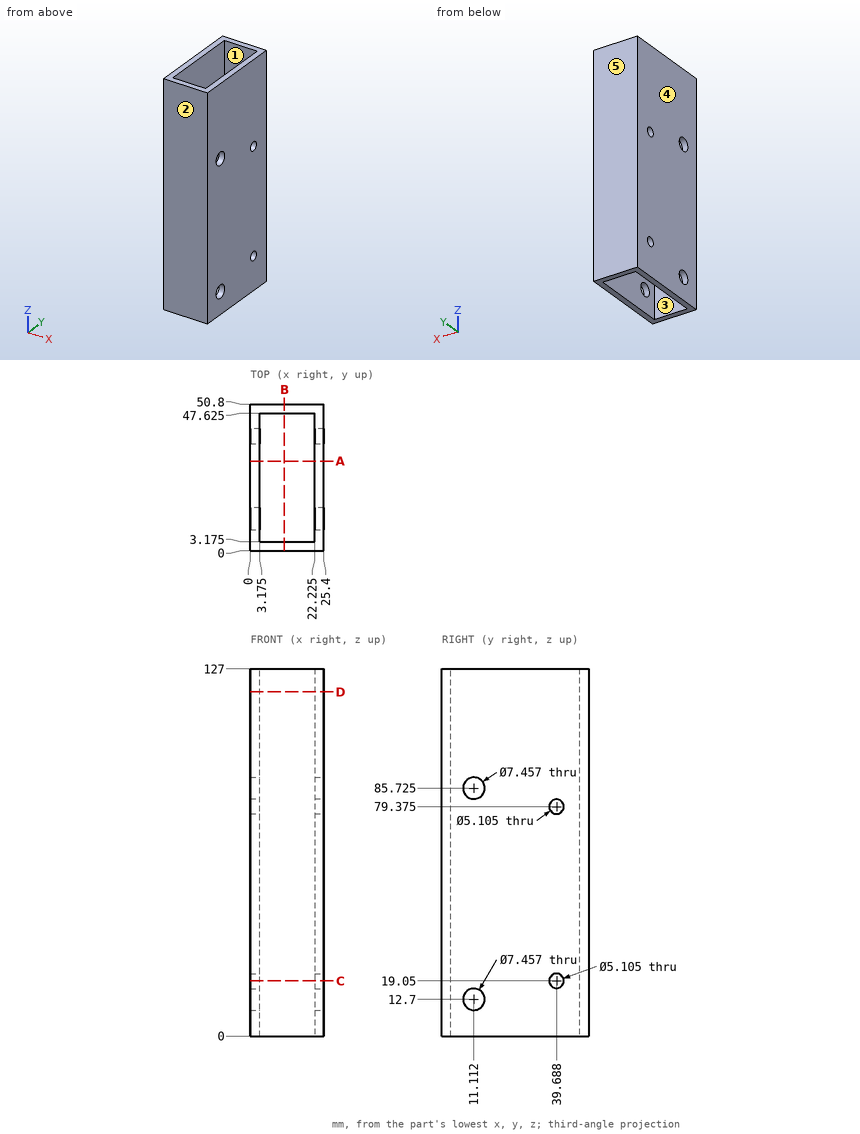
Source: three-view drawing plus pictorial views. Frame: mm from the lowest corner of the part. A direction names the side the tool comes from. Round coordinates to 2 decimals unless told otherwise and drop trailing zeros. Loops run counter-clockwise (first coordinate to the right, second up) from the corner with the lowest first, then second, coordinate; pieces in that order, holes last.
1. Section query A-A on y = 31. Output: boundary loops of the cut face in (x, z) (1 decimal).
2. Contact query for flat-ended pins moving along their axis: pin 1 (4.5 mm diameter, centred on y = 11.11, z = 85.72, fed in from +X); pin 2 (12 mm diameter, centred on x = 7.5, z = 35, fed in from -Y). Output: stop coordinate, or through.
3. Section query D-D on z = 119. Output: boundary loops of the cut face in (x, y) (1 decimal).
4. Mould query, pull axis X, two halves, no side actions, for the marked faces 3, 4 and 5. Classes: released by +X, released by -X, zero draft, split by the parting line, or undercut.
5. Ray query, L1, parallel to X at y = 31, z = 8 (1 decimal); L2, parallel to Y at x = 17.75, z = 112 (1 decimal). Return the intervals inside material, ascending.
6. Section query B-B on x = 11.75. Output: boundary loops of the cut face in (y, z) (1 decimal).
7. Access query for the marked faces 1 and 2. Directions: +Z, -Z, +X, -X, +Y, -Y. A direction counts if a zero-diameter tool reaches every point of the face in a straight line with its end or side. Return the directions, or none.
8. Section query C-C on z = 19.05. Output: boundary loops of the cut face in (x, y) (1 decimal).
Answers below:
1. outline: (0, 0) - (3.2, 0) - (3.2, 127) - (0, 127) - close; (22.2, 0) - (25.4, 0) - (25.4, 127) - (22.2, 127) - close
2. pin 1: passes through
2. pin 2: stops at y = 0
3. outline: (0, 0) - (25.4, 0) - (25.4, 50.8) - (0, 50.8) - close; hole (3.2, 3.2) - (22.2, 3.2) - (22.2, 47.6) - (3.2, 47.6) - close
4. face 3: undercut
4. face 4: released by -X
4. face 5: zero draft
5. L1: x = 0 to 3.2, 22.2 to 25.4
5. L2: y = 0 to 3.2, 47.6 to 50.8
6. outline: (0, 0) - (3.2, 0) - (3.2, 127) - (0, 127) - close; (47.6, 0) - (50.8, 0) - (50.8, 127) - (47.6, 127) - close
7. face 1: +Z, -Z
7. face 2: +Z, -Z, +X, -X, -Y
8. outline: (0, 0) - (25.4, 0) - (25.4, 37.1) - (22.2, 37.1) - (22.2, 3.2) - (3.2, 3.2) - (3.2, 37.1) - (0, 37.1) - close; (0, 42.2) - (3.2, 42.2) - (3.2, 47.6) - (22.2, 47.6) - (22.2, 42.2) - (25.4, 42.2) - (25.4, 50.8) - (0, 50.8) - close
